Geometry: see drawing. Coordinates: mm, zero at the bounding-box minimum. Give positions to 0.01 mm unless a question says otherwise; leave off trailing zeros. Loops run counter-clockwise (first coordinate to the right, second up) from the corner with the lowest first, then second, coordinate; pieces in that order, holes last. Notation, with made-up numbers: M -31,22 L 28,22 A25 cw 28,40 Z; hole C -2.75,84.25 d3. An arc over 180 degrees is marked long. Put each result on its own line as item: value.
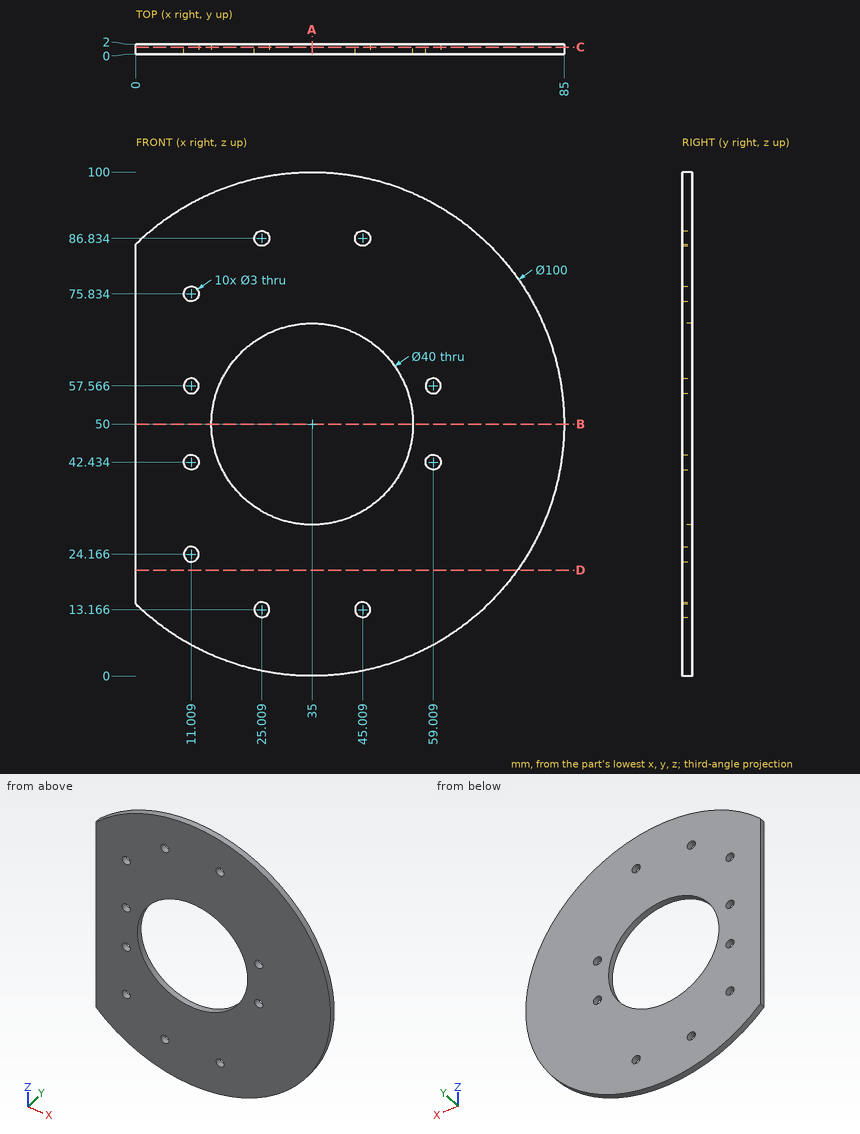
1. Section query A-A (x = 35). Output: boundary loops of the cut face in (y, z).
Found:
outline: M 0,0 L 2,0 L 2,30 L 0,30 Z; M 0,70 L 2,70 L 2,100 L 0,100 Z
2. Section query B-B (z = 50). Output: boundary loops of the cut face in (x, y).
Found:
outline: M 0,0 L 15,0 L 15,2 L 0,2 Z; M 55,0 L 85,0 L 85,2 L 55,2 Z
3. Section query C-C (y = 1.4). State how many separate pieces and enclosed holes the cut face has, plus the area to 3 significant figures.
Found:
separate pieces: 1
enclosed holes: 11
area: 5,790 mm^2
4. Section query D-D (z = 21). Output: boundary loops of the cut face in (x, y).
Found:
outline: M 0,0 L 75.73,0 L 75.73,2 L 0,2 Z
5. Material intervals for line 1 (Z direction, x = 11, y = 0.35) (1 decimal); line 2 (Z direction, x = 35, y = 0.8); line 3 (X direction, y = 0.75, z = 56.5) (1 decimal), sorted ascending. Write a range as from..to.
Found:
line 1: 6.1..22.7, 25.7..40.9, 43.9..56.1, 59.1..74.3, 77.3..93.9
line 2: 0..30, 70..100
line 3: 0..10, 12.1..16.1, 53.9..58, 60.1..84.6
6. Contact query for flat-ended pins moving along their axis: P1, Ø4, axis at x = 25.01, z = 86.83, coming from the +Y side; P2, Ø2.5, axis at x = 45.01, z = 13.17, coming from the -Y side. Output: stop coordinate, or through.
Found:
P1: y = 2
P2: through
